from build123d import *

# Parameters (mm, degrees)
BRIDA_BASE2_DEPTH                = 1.5
BRIDA_DE_ARISTA3_STRIP_W         = 8
BRIDA_DE_ARISTA3_STRIP_H         = 1.5
BRIDA_DE_ARISTA3_STRIP_CUT_DEPTH = 40
BRIDA_DE_ARISTA3_DEPTH           = 40
BRIDA_DE_ARISTA4_STRIP_W         = 8
BRIDA_DE_ARISTA4_STRIP_H         = 1.5
BRIDA_DE_ARISTA4_STRIP_CUT_DEPTH = 9
BRIDA_DE_ARISTA4_DEPTH           = 9
BRIDA_DE_ARISTA5_STRIP_W         = 8
BRIDA_DE_ARISTA5_STRIP_H         = 1.5
BRIDA_DE_ARISTA5_STRIP_CUT_DEPTH = 9
BRIDA_DE_ARISTA5_DEPTH           = 9
REDONDEO1_R                      = 5
REDONDEO2_R                      = 5
REDONDEO3_R                      = 5
REDONDEO4_R                      = 5
REDONDEO5_R                      = 5
REDONDEO6_R                      = 5
REDONDEO7_R                      = 5
REDONDEO8_R                      = 5
CROQUIS39_R                      = 4
CORTAR_EXTRUIR2_DEPTH            = 2
CROQUIS40_R                      = 1.5
CORTAR_EXTRUIR3_DEPTH            = 2
MATRIZC1_COUNT                   = 4
CROQUIS41_R                      = 1.5
CORTAR_EXTRUIR4_DEPTH            = 2
MATRIZC2_COUNT                   = 4
CROQUIS42_R                      = 1.5
CORTAR_EXTRUIR5_DEPTH            = 2
MATRIZC3_COUNT                   = 4
CROQUIS46_R                      = 2
CORTAR_EXTRUIR9_DEPTH            = 2
CROQUIS49_R                      = 2
CORTAR_EXTRUIR10_DEPTH           = 2
CROQUIS51_R                      = 1.500000001
CORTAR_EXTRUIR11_DEPTH           = 2
CROQUIS52_R                      = 1.500000001
CORTAR_EXTRUIR12_DEPTH           = 2
CROQUIS53_R                      = 1.500000001
CORTAR_EXTRUIR13_DEPTH           = 2
MATRIZC4_COUNT                   = 4
MATRIZC5_COUNT                   = 4


# Sheet-metal steps are written as plain solids
with BuildPart() as part:
    # Croquis1 → Brida base2 (new body)
    with BuildSketch(Plane.XY):
        Polygon((20, -17.745), (20, -12.745), (29, -12.745), (29, 10.755), (20, 10.755), (20, 7.745), (19, 7.745), (19, 17.745), (-19, 17.745), (-19, 7.745), (-20, 7.745), (-20, 10.755), (-29, 10.755), (-29, -12.745), (-20, -12.745), (-20, -17.745), align=None)
    extrude(amount=-BRIDA_BASE2_DEPTH)

    # Brida de arista3 strip (across the edge) → Brida de arista3 strip cut (cut)
    with BuildSketch(Plane(origin=(-20, -17.745, 0), x_dir=(0, 1, 0), z_dir=(1, 0, 0))):
        with Locations((-3, -0.75)):
            Rectangle(BRIDA_DE_ARISTA3_STRIP_W, BRIDA_DE_ARISTA3_STRIP_H)
    extrude(amount=BRIDA_DE_ARISTA3_STRIP_CUT_DEPTH, mode=Mode.SUBTRACT)

    # Brida de arista3 section (across the edge) → Brida de arista3 (add)
    with BuildSketch(Plane(origin=(-20, -17.745, 0), x_dir=(0, 1, 0), z_dir=(1, 0, 0))):
        with BuildLine():
            Line((-1.5, 1), (-1.5, 24.5))
            Line((-1.5, 24.5), (0, 24.5))
            Line((0, 24.5), (0, 1))
            ThreePointArc((0, 1), (0.292893219, 0.292893219), (1, 0))
            Line((1, 0), (1, -1.5))
            ThreePointArc((1, -1.5), (-0.767766953, -0.767766953), (-1.5, 1))
        make_face()
    extrude(amount=BRIDA_DE_ARISTA3_DEPTH)

    # Brida de arista4 strip (across the edge) → Brida de arista4 strip cut (cut)
    with BuildSketch(Plane(origin=(29, 10.755, 0), x_dir=(0, -1, 0), z_dir=(-1, 0, 0))):
        with Locations((-3, -0.75)):
            Rectangle(BRIDA_DE_ARISTA4_STRIP_W, BRIDA_DE_ARISTA4_STRIP_H)
    extrude(amount=BRIDA_DE_ARISTA4_STRIP_CUT_DEPTH, mode=Mode.SUBTRACT)

    # Brida de arista4 section (across the edge) → Brida de arista4 (add)
    with BuildSketch(Plane(origin=(29, 10.755, 0), x_dir=(0, -1, 0), z_dir=(-1, 0, 0))):
        with BuildLine():
            Line((-1.5, 1), (-1.5, 24.5))
            Line((-1.5, 24.5), (0, 24.5))
            Line((0, 24.5), (0, 1))
            ThreePointArc((0, 1), (0.292893219, 0.292893219), (1, 0))
            Line((1, 0), (1, -1.5))
            ThreePointArc((1, -1.5), (-0.767766953, -0.767766953), (-1.5, 1))
        make_face()
    extrude(amount=BRIDA_DE_ARISTA4_DEPTH)

    # Brida de arista5 strip (across the edge) → Brida de arista5 strip cut (cut)
    with BuildSketch(Plane(origin=(-20, 10.755, 0), x_dir=(0, -1, 0), z_dir=(-1, 0, 0))):
        with Locations((-3, -0.75)):
            Rectangle(BRIDA_DE_ARISTA5_STRIP_W, BRIDA_DE_ARISTA5_STRIP_H)
    extrude(amount=BRIDA_DE_ARISTA5_STRIP_CUT_DEPTH, mode=Mode.SUBTRACT)

    # Brida de arista5 section (across the edge) → Brida de arista5 (add)
    with BuildSketch(Plane(origin=(-20, 10.755, 0), x_dir=(0, -1, 0), z_dir=(-1, 0, 0))):
        with BuildLine():
            Line((-1.5, 1), (-1.5, 24.5))
            Line((-1.5, 24.5), (0, 24.5))
            Line((0, 24.5), (0, 1))
            ThreePointArc((0, 1), (0.292893219, 0.292893219), (1, 0))
            Line((1, 0), (1, -1.5))
            ThreePointArc((1, -1.5), (-0.767766953, -0.767766953), (-1.5, 1))
        make_face()
    extrude(amount=BRIDA_DE_ARISTA5_DEPTH)

    # Redondeo1
    redondeo1_edges = [part.edges().sort_by_distance(p)[0] for p in [
        (19, 17.745, -0.75),
    ]]
    fillet(redondeo1_edges, radius=REDONDEO1_R)

    # Redondeo2
    redondeo2_edges = [part.edges().sort_by_distance(p)[0] for p in [
        (-19, 17.745, -0.75),
    ]]
    fillet(redondeo2_edges, radius=REDONDEO2_R)

    # Redondeo3
    redondeo3_edges = [part.edges().sort_by_distance(p)[0] for p in [
        (-29, -12.745, -0.75),
    ]]
    fillet(redondeo3_edges, radius=REDONDEO3_R)

    # Redondeo4
    redondeo4_edges = [part.edges().sort_by_distance(p)[0] for p in [
        (29, -12.745, -0.75),
    ]]
    fillet(redondeo4_edges, radius=REDONDEO4_R)

    # Redondeo5
    redondeo5_edges = [part.edges().sort_by_distance(p)[0] for p in [
        (20, -18.495, 24.5),
    ]]
    fillet(redondeo5_edges, radius=REDONDEO5_R)

    # Redondeo6
    redondeo6_edges = [part.edges().sort_by_distance(p)[0] for p in [
        (-20, -18.495, 24.5),
    ]]
    fillet(redondeo6_edges, radius=REDONDEO6_R)

    # Redondeo7
    # the kernel refuses this fillet: 5 mm, written as the material it takes off along each edge
    with BuildSketch(Plane(origin=(20, 24.755, 24.5), x_dir=(0, 0, -1), z_dir=(0, -1, 0))) as redondeo7_piece_1:
        with BuildLine():
            CenterArc((REDONDEO7_R, REDONDEO7_R), REDONDEO7_R, 180, 90)
            Line((0, REDONDEO7_R), (0, 0))
            Line((0, 0), (REDONDEO7_R, 0))
        make_face()
    extrude(amount=26.5, mode=Mode.SUBTRACT)
    with BuildSketch(Plane(origin=(29, 24.755, 24.5), x_dir=(0, 0, -1), z_dir=(0, -1, 0))) as redondeo7_piece_2:
        with BuildLine():
            CenterArc((REDONDEO7_R, -REDONDEO7_R), REDONDEO7_R, 90, 90)
            Line((0, -REDONDEO7_R), (0, 0))
            Line((0, 0), (REDONDEO7_R, 0))
        make_face()
    extrude(amount=26.5, mode=Mode.SUBTRACT)

    # Redondeo8
    # the kernel refuses this fillet: 5 mm, written as the material it takes off along each edge
    with BuildSketch(Plane(origin=(-29, 24.755, 24.5), x_dir=(0, 0, -1), z_dir=(0, -1, 0))) as redondeo8_piece_1:
        with BuildLine():
            CenterArc((REDONDEO8_R, REDONDEO8_R), REDONDEO8_R, 180, 90)
            Line((0, REDONDEO8_R), (0, 0))
            Line((0, 0), (REDONDEO8_R, 0))
        make_face()
    extrude(amount=26.5, mode=Mode.SUBTRACT)
    with BuildSketch(Plane(origin=(-20, 24.755, 24.5), x_dir=(0, 0, -1), z_dir=(0, -1, 0))) as redondeo8_piece_2:
        with BuildLine():
            CenterArc((REDONDEO8_R, -REDONDEO8_R), REDONDEO8_R, 90, 90)
            Line((0, -REDONDEO8_R), (0, 0))
            Line((0, 0), (REDONDEO8_R, 0))
        make_face()
    extrude(amount=26.5, mode=Mode.SUBTRACT)

    # Croquis39 → Cortar-Extruir2 (cut)
    with BuildSketch(Plane.XY):
        with Locations((-10.5, 4.755)):
            Circle(CROQUIS39_R)
        with Locations((10.5, 4.755)):
            Circle(CROQUIS39_R)
        with Locations((0, -5.745)):
            Circle(CROQUIS39_R)
    extrude(amount=-CORTAR_EXTRUIR2_DEPTH, mode=Mode.SUBTRACT)

    # Croquis40 → Cortar-Extruir3 (cut)
    with BuildSketch(Plane.XY):
        with Locations((-10.5, 11.755)):
            Circle(CROQUIS40_R)
    cortar_extruir3 = extrude(amount=-CORTAR_EXTRUIR3_DEPTH, mode=Mode.SUBTRACT)

    # MatrizC1: Cortar-Extruir3 ×4 about axis
    matrizc1_axis = Axis((-10.5, 4.755, 0), (0, 0, 1))
    for i in range(1, MATRIZC1_COUNT):
        add(cortar_extruir3.rotate(matrizc1_axis, i * 360 / MATRIZC1_COUNT), mode=Mode.SUBTRACT)

    # Croquis41 → Cortar-Extruir4 (cut)
    with BuildSketch(Plane.XY):
        with Locations((0, 1.255)):
            Circle(CROQUIS41_R)
    cortar_extruir4 = extrude(amount=-CORTAR_EXTRUIR4_DEPTH, mode=Mode.SUBTRACT)

    # MatrizC2: Cortar-Extruir4 ×4 about axis
    matrizc2_axis = Axis((0, -5.745, 0), (0, 0, 1))
    for i in range(1, MATRIZC2_COUNT):
        add(cortar_extruir4.rotate(matrizc2_axis, i * 360 / MATRIZC2_COUNT), mode=Mode.SUBTRACT)

    # Croquis42 → Cortar-Extruir5 (cut)
    with BuildSketch(Plane.XY):
        with Locations((10.5, 11.755)):
            Circle(CROQUIS42_R)
    cortar_extruir5 = extrude(amount=-CORTAR_EXTRUIR5_DEPTH, mode=Mode.SUBTRACT)

    # MatrizC3: Cortar-Extruir5 ×4 about axis
    matrizc3_axis = Axis((10.5, 4.755, 0), (0, 0, 1))
    for i in range(1, MATRIZC3_COUNT):
        add(cortar_extruir5.rotate(matrizc3_axis, i * 360 / MATRIZC3_COUNT), mode=Mode.SUBTRACT)

    # Croquis46 → Cortar-Extruir9 (cut)
    with BuildSketch(Plane.XY):
        with Locations((24, 3.755)):
            Circle(CROQUIS46_R)
        with Locations((24, -6.245)):
            Circle(CROQUIS46_R)
        with Locations((-24, 3.755)):
            Circle(CROQUIS46_R)
        with Locations((-24, -6.245)):
            Circle(CROQUIS46_R)
    extrude(amount=-CORTAR_EXTRUIR9_DEPTH, mode=Mode.SUBTRACT)

    # Croquis49 → Cortar-Extruir10 (cut)
    with BuildSketch(Plane(origin=(0, 12.255, 0), x_dir=(1, 0, 0), z_dir=(0, 1, 0))):
        with Locations(Location((-24, -7.199489743, 0), (0, 0, 270))):
            Circle(CROQUIS49_R)
        with Locations(Location((24, -7.199489743, 0), (0, 0, 270))):
            Circle(CROQUIS49_R)
        with Locations(Location((24, -17.199489743, 0), (0, 0, 270))):
            Circle(CROQUIS49_R)
        with Locations(Location((-24, -17.199489743, 0), (0, 0, 270))):
            Circle(CROQUIS49_R)
    extrude(amount=-CORTAR_EXTRUIR10_DEPTH, mode=Mode.SUBTRACT)

    # Croquis51 → Cortar-Extruir11 (cut)
    with BuildSketch(Plane(origin=(0, -17.745, 0), x_dir=(1, 0, 0), z_dir=(0, 1, 0))):
        with Locations(Location((-10, -12.199489743, 0), (0, 0, 270))):
            Circle(CROQUIS51_R)
        with Locations(Location((10, -12.199489743, 0), (0, 0, 270))):
            Circle(CROQUIS51_R)
    extrude(amount=-CORTAR_EXTRUIR11_DEPTH, mode=Mode.SUBTRACT)

    # Croquis52 → Cortar-Extruir12 (cut)
    with BuildSketch(Plane(origin=(0, -17.745, 0), x_dir=(1, 0, 0), z_dir=(0, 1, 0))):
        with Locations(Location((-10, -5.199489743, 0), (0, 0, 270))):
            Circle(CROQUIS52_R)
    cortar_extruir12 = extrude(amount=-CORTAR_EXTRUIR12_DEPTH, mode=Mode.SUBTRACT)

    # Croquis53 → Cortar-Extruir13 (cut)
    with BuildSketch(Plane(origin=(0, -17.745, 0), x_dir=(1, 0, 0), z_dir=(0, 1, 0))):
        with Locations(Location((10, -5.199489743, 0), (0, 0, 270))):
            Circle(CROQUIS53_R)
    cortar_extruir13 = extrude(amount=-CORTAR_EXTRUIR13_DEPTH, mode=Mode.SUBTRACT)

    # MatrizC4: Cortar-Extruir12 ×4 about axis
    matrizc4_axis = Axis((-10, 0, 12.199489743), (0, 1, 0))
    for i in range(1, MATRIZC4_COUNT):
        add(cortar_extruir12.rotate(matrizc4_axis, i * 360 / MATRIZC4_COUNT), mode=Mode.SUBTRACT)

    # MatrizC5: Cortar-Extruir13 ×4 about axis
    matrizc5_axis = Axis((10, 0, 12.199489743), (0, 1, 0))
    for i in range(1, MATRIZC5_COUNT):
        add(cortar_extruir13.rotate(matrizc5_axis, i * 360 / MATRIZC5_COUNT), mode=Mode.SUBTRACT)


solid = part.part
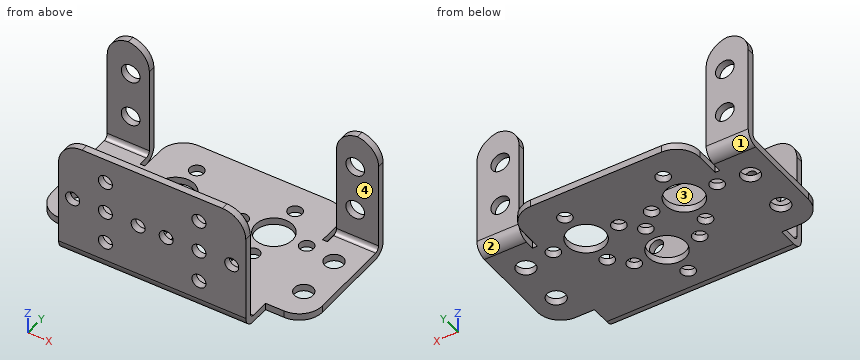
Check sheet for the modelled part. Datum: model origin and axes. Units: mm. Face numbers are marked on the shaded views. A direction names the side the tool comes from. Round coordinates to 2 decimals unless told otherwise and drop trailing zeros. Loops run counter-clockwise (first coordinate to the right, second up) from the corner with the lowest first, then second, coordinate; pieces in that order, holes last. Notation, with made-up numbers: (3.5, 88.5) -> (32.5, 88.5) arc R9 cw to (32.5, 95.5) -> close; hole circle Ø7 at (-5, 6). An arc over 180 degrees is marked (long way). Put each result on its own line as item: value. Start each with the question number.
1. Access from +Z, -Z, +X, -X, +Y, -Y to the whole of each face (thin tool, end or side, straight path). Record for the marked faces 1, 2, 3 and 4.
2. Gauge pin test, flat ends, axial feed: pin 1 (10 mm diameter, centred on x = -16, z = 1.5, fed in from +Y) (3 decimals); pin 2 (4 mm diameter, centred on x = -13.5, y = -1, fed in from +Z); pin 3 (5 mm diameter, centred on x = 24, z = 7.2, fed in from +Y) (3 decimals); pin 4 (0.8 mm diameter, centred on x = -19.5, z = -0.5, fed in from +Y) (3 decimals). Record the tip position at first contact, or that the pin passes through.
3. Section check C-C (x = -17.5). Enter the section's corners in (y, z) (3 decimals), plus the area to 3 significant figures.
4. Section check A-A (z = 4.5). Enter the section's corners in (x, y) (3 decimals).
5. Section check B-B (x = 10). Give the number of separate pieces and of enclosed holes in the cut face, plus the area to 3 significant figures.
6. Scan lines: probe 1 along Y at (x, z) = (-8, 11.5) (3 decimals); probe 2 along Z at (x, y) = (14.5, -0.5); probe 3 along Y at (x, z) = (-24.5, 5) (3 decimals). Record each from-to range of solid material in increasing order.
Findings:
1. face 1: -Z, -X, +Y
1. face 2: -Z, +X, +Y
1. face 3: +Z, +X, -X, +Y
1. face 4: +Z, +X, -X, -Y
2. pin 1: stops at y = 17.745
2. pin 2: stops at z = 0
2. pin 3: stops at y = 12.255
2. pin 4: stops at y = 7.745
3. outline: (-19.245, 1) arc R2.5 ccw to (-16.745, -1.5) -> (3.255, -1.5) -> (3.255, 0) -> (-16.745, 0) arc R1 cw to (-17.745, 1) -> (-17.745, 10.785) -> (-19.245, 10.785) -> close; (-19.245, 13.614) -> (-17.745, 13.614) -> (-17.745, 23.83) -> (-19.245, 23.83) -> close; (6.255, -1.5) -> (16.316, -1.5) -> (16.316, 0) -> (6.255, 0) -> close
3. area: 79.2 mm^2
4. outline: (-29, 10.755) -> (-20, 10.755) -> (-20, 12.255) -> (-29, 12.255) -> close; (-20, -19.245) -> (-11.327, -19.245) -> (-11.327, -17.745) -> (-20, -17.745) -> close; (-8.673, -19.245) -> (8.673, -19.245) -> (8.673, -17.745) -> (-8.673, -17.745) -> close; (11.327, -19.245) -> (20, -19.245) -> (20, -17.745) -> (11.327, -17.745) -> close; (20, 10.755) -> (29, 10.755) -> (29, 12.255) -> (20, 12.255) -> close
5. separate pieces: 7
5. enclosed holes: 0
5. area: 57.2 mm^2
6. probe 1: y = -19.245 to -17.745
6. probe 2: z = -1.5 to 0
6. probe 3: y = 10.755 to 12.255
